Autodesk Inventor part; units mm, degrees
ref_plane "YZ Plane" through (0, 0, 0) normal (1, 0, 0) x (0, 1, 0)
ref_plane "XZ Plane" through (0, 0, 0) normal (0, 1, 0) x (-1, 0, 0)
ref_plane "XY Plane" through (0, 0, 0) normal (0, 0, 1) x (1, 0, 0)
sketch "Sketch1" plane through (0, 0, 0) normal (0, 1, 0) x (-1, 0, 0)
  line L0 (-37.5, 27.5) -> (37.5, 27.5)
  line L1 (37.5, 27.5) -> (37.5, -27.5)
  line L2 (37.5, -27.5) -> (-37.5, -27.5)
  line L3 (-37.5, -27.5) -> (-37.5, 27.5)
  line L4 (-37.5, 27.5) -> (37.5, -27.5) construction
  line L5 (37.5, 27.5) -> (-37.5, -27.5) construction
  circle A0 centre (27.5, -18.5) radius 5.5
  circle A1 centre (-27.5, -18.5) radius 5.5
  circle A2 centre (0, 19.5) radius 7.5
  circle A3 centre (10.5, 4.5) radius 7.5
  circle A4 centre (-10.5, 4.5) radius 7.5
  point P0 (0, 0)
  point P1 (0, 27.5)
  dimension "d0" = 75
  dimension "d1" = 55
  dimension "d2" = 11
  dimension "d4" = 11
  dimension "d6" = 55
  dimension "d7" = 10
  dimension "d8" = 10
  dimension "d9" = 15
  dimension "d11" = 15
  dimension "d13" = 15
  dimension "d15" = 23
  dimension "d16" = 8
  dimension "d17" = 21
  dimension "d18" = 10.5
  dimension "d19" = 46
extrude "Extrusion1" add sketch "Sketch1" along normal blind 7
sketch "Sketch2" plane through (0, 7, 0) normal (0, 1, 0) x (1, 0, 0)
  line L0 (37.5, 27.5) -> (-37.5, 27.5)
  line L1 (37.5, -27.5) -> (-37.5, -27.5)
  line L2 (-37.5, -27.5) -> (-37.5, 27.5)
  line L3 (-37.5, 27.5) -> (37.5, 27.5)
  line L4 (37.5, 27.5) -> (37.5, -27.5)
  line L5 (37.5, -27.5) -> (-37.5, 27.5) construction
  line L6 (-37.5, -27.5) -> (37.5, 27.5) construction
  circle A0 centre (-27.5, 18.5) radius 3
  circle A1 centre (27.5, 18.5) radius 3
  circle A2 centre (-10.5, -4.5) radius 7.5
  circle A3 centre (10.5, -4.5) radius 7.5
  circle A4 centre (0, -19.5) radius 7.5
  circle A5 centre (0, -19.5) radius 4
  circle A6 centre (-10.5, -4.5) radius 4
  circle A7 centre (10.5, -4.5) radius 4
  line L7 (-37.5, -27.5) -> (37.5, -27.5)
  point P0 (0, 0)
  point P1 (0, -27.5)
  point P2 (0, -27.5)
  dimension "d22" = 6
  dimension "d23" = 6
  dimension "d24" = 15
  dimension "d25" = 15
  dimension "d26" = 15
  dimension "d27" = 8
  dimension "d28" = 8
  dimension "d29" = 8
  dimension "d30" = 55
  dimension "d31" = 10
  dimension "d32" = 10
  dimension "d33" = 46
  dimension "d34" = 23
  dimension "d35" = 8
  dimension "d36" = 10.5
  dimension "d37" = 10.5
  dimension "d38" = 21
extrude "Extrusion2" add sketch "Sketch2" along normal blind 3 contours L4 L1 L2 L0
sketch "Sketch3" plane through (0, 10, 0) normal (0, 1, 0) x (1, 0, 0)
  line L0 (37.5, 27.5) -> (-37.5, 27.5)
  line L1 (37.5, -27.5) -> (-37.5, -27.5)
  line L2 (-37.5, -27.5) -> (-37.5, 27.5)
  line L3 (-37.5, 27.5) -> (37.5, 27.5)
  line L4 (37.5, 27.5) -> (37.5, -27.5)
  line L5 (37.5, -27.5) -> (-37.5, 27.5) construction
  line L6 (-37.5, -27.5) -> (37.5, 27.5) construction
  circle A0 centre (-27.5, 18.5) radius 3
  circle A1 centre (-27.5, 18.5) radius 3
  circle A2 centre (27.4955, 18.5) radius 3
  circle A3 centre (-10.5, -4.5) radius 4
  circle A4 centre (10.5, -4.5) radius 4
  circle A5 centre (0, -19.5) radius 4
  line L7 (-37.5, -27.5) -> (37.5, -27.5)
  point P0 (0, 0)
  point P1 (0, -27.5)
  point P2 (0, -27.5)
  dimension "d41" = 6
  dimension "d42" = 8
  dimension "d43" = 8
  dimension "d44" = 8
  dimension "d45" = 8
  dimension "d46" = 23
  dimension "d47" = 10.5
  dimension "d48" = 10.5
extrude "Extrusion3" add sketch "Sketch3" along normal blind 8
sketch "Sketch4" plane through (0, 18, 0) normal (0, 1, 0) x (1, 0, 0)
  line L0 (-37.5, 8.5) -> (37.5, 8.5)
  line L1 (-37.5, -27.5) -> (37.5, -27.5)
  line L2 (-37.5, 27.5) -> (-37.5, -27.5)
  line L3 (-37.5, 8.5) -> (-37.5, -27.5)
  line L4 (-37.5, -27.5) -> (37.5, -27.5)
  line L5 (-37.5, -27.5) -> (37.5, -27.5)
  line L6 (37.5, -27.5) -> (37.5, 8.5)
  circle A0 centre (-10.5, -4.5) radius 4
  circle A1 centre (10.5, -4.5) radius 4
  circle A2 centre (0, -19.5) radius 4
  point P0 (0, 0)
  point P1 (0, -27.5)
  dimension "d51" = 75
  dimension "d52" = 36
  dimension "d53" = 8
  dimension "d54" = 8
  dimension "d55" = 8
  dimension "d56" = 8
  dimension "d57" = 23
  dimension "d58" = 21
  dimension "d59" = 10.5
extrude "Extrusion4" add sketch "Sketch4" along normal blind 7
properties part number "Feste Backe" material "Steel"
Here's how the part is built. I have some questions about the finished solid (model axes, mm). A direction names the side the tool comes from. Round coordinates to 2 decimals unless told otherwise and drop trailing zeros. Order: outer loops, then holes, each group sorted by start corner. A loop starts at its lowest first (then second) coordinate and runs counter-clockwise, first axis right, second up. Notation, with made-up numbers: M 62.5,80 L 104.5,80 A19 cw 104.5,87 Z; hole C -15,33 d3. An arc over 180 degrees is marked long. Answer in a Markdown table with one row per item.
Item 1: I'm going to push flat-ended pins straight in: pin 1 (3.5 mm diameter, centred on x = 29.5, z = -19.5, fed in from -Y); pin 2 (7 mm diameter, centred on x = -10.5, z = 4.5, fed in from +Y); pin 3 (12 mm diameter, centred on x = -10.5, z = 4.5, fed in from -Y); pin 4 (10 mm diameter, centred on x = -23.5, z = -14, fed in from +Y). Where does each tip first touch, or does it pass through?
A:
| item | result |
|---|---|
| pin 1 | stops at y = 7 |
| pin 2 | passes through |
| pin 3 | stops at y = 10 |
| pin 4 | stops at y = 18 |
Item 2: Imagine slicing it at B-B, the plane x = -27.5. Write out the boundary of the cut face in (y, z).
A:
| item | result |
|---|---|
| outline | M 0,-27.5 L 18,-27.5 L 18,-21.5 L 7,-21.5 L 7,-24 L 0,-24 Z; M 0,-13 L 7,-13 L 7,-15.5 L 18,-15.5 L 18,-8.5 L 25,-8.5 L 25,27.5 L 0,27.5 Z |
Item 3: Imagine slicing it at D-D, the plane z = 1.5. Write out the boundary of the cut face in (x, y), and give its area (3 significant figures).
A:
| item | result |
|---|---|
| outline | M -37.5,0 L -17.37,0 L -17.37,10 L -13.15,10 L -13.15,25 L -37.5,25 Z; M -7.85,10 L -3.63,10 L -3.63,0 L 3.63,0 L 3.63,10 L 7.85,10 L 7.85,25 L -7.85,25 Z; M 13.15,10 L 17.37,10 L 17.37,0 L 37.5,0 L 37.5,25 L 13.15,25 Z |
| area | 1,440 mm2 |
Item 4: Imagine slicing it at A-A, the plane y = 3.5. Write out the boundary of the cut face in (x, z).
A:
| item | result |
|---|---|
| outline | M -37.5,-27.5 L 37.5,-27.5 L 37.5,27.5 L -37.5,27.5 Z; hole C -27.5,-18.5 d11; hole C -10.5,4.5 d15; hole C 0,19.5 d15; hole C 10.5,4.5 d15; hole C 27.5,-18.5 d11 |
Item 5: Thinking about a two-plate mould opening in Z: for faces 4 (the face through (1, 9, -27.5)), 5 (the face through (37.5, 12, 0)), 6 (the face through (7.3, 17.4, 2.1)), which applies, +Z half, -Z half, draft (parallel to the pull), parting line (faces both ways), or undercut?
A:
| item | result |
|---|---|
| face 4 | -Z half |
| face 5 | draft |
| face 6 | undercut |
Item 6: For faces 1 (the face through (-37.5, 12, 0)), 2 (the face through (-1, 18, -18)), 3 (the face through (-23.45, 3.45, -22.22)), which set-ups out of +Z, -Z, +X, -X, +Y, -Y let a thin tool reach every point of the face, with its end or its side?
A:
| item | result |
|---|---|
| face 1 | +Z, -Z, -X, +Y, -Y |
| face 2 | -Z, +X, -X, +Y |
| face 3 | -Y |
Item 7: If I drill on L1, parallel to X at y = 14.25, z = 4.5; L2, parallel to Z at x = -27.5, y = 12.75; L3, parallel to X at y = 8.65, z = -18.5, over which ranges is the centre line in solid material (lowest first)? Write a range as from..to.
A:
| item | result |
|---|---|
| L1 | x = -37.5..-14.5, -6.5..6.5, 14.5..37.5 |
| L2 | z = -27.5..-21.5, -15.5..27.5 |
| L3 | x = -37.5..-30.5, -24.5..24.5, 30.5..37.5 |
